from build123d import *

# Parameters (mm, degrees)
SKETCH_8_W               = 220
SKETCH_8_H               = 120
EXTRUDE_6_DEPTH          = 3
SKETCH_10_W              = 10
SKETCH_10_H              = 120
EXTRUDE_7_DEPTH          = 27
CUT_EXTRUDE_1_DEPTH      = 129.175660716
CUT_EXTRUDE_1_DEPTH_BACK = 129.175660716
SKETCH_9_R               = 2.05
SKETCH_11_R              = 3.6
CUT_EXTRUDE_2_DEPTH      = 25
CUT_EXTRUDE_4_DEPTH      = 129.175660716
CUT_EXTRUDE_4_DEPTH_BACK = 129.175660716
SKETCH_13_W              = 40
SKETCH_13_H              = 18.5
SKETCH_14_W              = 140
SKETCH_14_H              = 44
CUT_EXTRUDE_7_DEPTH      = 1
SKETCH_15_W              = 15
SKETCH_15_H              = 80
SKETCH_15_H_2            = 40
SKETCH_15_W_2            = 30
SKETCH_15_H_3            = 16
CUT_EXTRUDE_8_DEPTH      = 129.840987267
SKETCH_9_5_R             = 2
CUT_EXTRUDE_9_DEPTH      = 129.175660716
CUT_EXTRUDE_13_DEPTH     = 27
SKETCH_20_W              = 135
SKETCH_20_H              = 8
EXTRUDE_8_DEPTH          = 2
FILLET_1_R               = 3
FILLET_2_R               = 2


with BuildPart() as part:
    # Sketch 8 → Extrude 6 (new body)
    with BuildSketch(Plane(origin=(0, 0, 0), x_dir=(1, 0, 0), z_dir=(0, 1, 0))):
        Rectangle(SKETCH_8_W, SKETCH_8_H)
    extrude(amount=EXTRUDE_6_DEPTH)

    # Sketch 10 → Extrude 7 (add)
    with BuildSketch(Plane.XZ):
        with Locations((-105, 0)):
            Rectangle(SKETCH_10_W, SKETCH_10_H)
        with Locations((105, 0)):
            Rectangle(SKETCH_10_W, SKETCH_10_H)
    extrude(amount=EXTRUDE_7_DEPTH)

    # Sketch 9 → Cut-Extrude 1 (cut, two sides: drawn at the far end of the back side and taken through both)
    with BuildSketch(Plane(origin=(0, 0, 0), x_dir=(1, 0, 0), z_dir=(0, 1, 0)).offset(-CUT_EXTRUDE_1_DEPTH_BACK)):
        with Locations(Location((104.5, 54.5, 0), (0, 0, 270))):
            Circle(SKETCH_9_R)
        with Locations(Location((-104.5, 54.5, 0), (0, 0, 90))):
            Circle(SKETCH_9_R)
        with Locations(Location((-104.5, -54.5, 0), (0, 0, 270))):
            Circle(SKETCH_9_R)
        with Locations(Location((104.5, -54.5, 0), (0, 0, 90))):
            Circle(SKETCH_9_R)
    extrude(amount=CUT_EXTRUDE_1_DEPTH + CUT_EXTRUDE_1_DEPTH_BACK, mode=Mode.SUBTRACT)

    # Sketch 11 → Cut-Extrude 2 (cut)
    with BuildSketch(Plane(origin=(0, 3, 0), x_dir=(1, 0, 0), z_dir=(0, 1, 0))):
        with Locations(Location((-104.497380754, 54.5, 0), (0, 0, 270))):
            Circle(SKETCH_11_R)
        with Locations(Location((-104.497380754, -54.5, 0), (0, 0, 90))):
            Circle(SKETCH_11_R)
        with Locations(Location((104.5, -54.5, 0), (0, 0, 270))):
            Circle(SKETCH_11_R)
        with Locations(Location((104.5, 54.5, 0), (0, 0, 90))):
            Circle(SKETCH_11_R)
    extrude(amount=-CUT_EXTRUDE_2_DEPTH, mode=Mode.SUBTRACT)

    # Sketch 13 → Cut-Extrude 4 (cut, two sides: drawn at the far end of the back side and taken through both)
    with BuildSketch(Plane(origin=(0, 0, 0), x_dir=(0, 0, -1), z_dir=(1, 0, 0)).offset(-CUT_EXTRUDE_4_DEPTH_BACK)):
        with Locations((-25, -12.75)):
            Rectangle(SKETCH_13_W, SKETCH_13_H)
        with Locations((25, -12.75)):
            Rectangle(SKETCH_13_W, SKETCH_13_H)
    extrude(amount=CUT_EXTRUDE_4_DEPTH + CUT_EXTRUDE_4_DEPTH_BACK, mode=Mode.SUBTRACT)

    # Sketch 14 → Cut-Extrude 7 (cut)
    with BuildSketch(Plane(origin=(0, 3, 0), x_dir=(1, 0, 0), z_dir=(0, 1, 0))):
        Rectangle(SKETCH_14_W, SKETCH_14_H)
    extrude(amount=-CUT_EXTRUDE_7_DEPTH, mode=Mode.SUBTRACT)

    # Sketch 15 → Cut-Extrude 8 (cut, through all)
    with BuildSketch(Plane(origin=(0, 3, 0), x_dir=(1, 0, 0), z_dir=(0, 1, 0))):
        with Locations((-92.5, 0)):
            Rectangle(SKETCH_15_W, SKETCH_15_H)
        with Locations((92.5, 25)):
            Rectangle(SKETCH_15_W, SKETCH_15_H_2)
        Polygon((-44.702941459, -12), (44.702941459, -12), (0, -3.059411708), align=None)
        Polygon((-60, -8.940588292), (-60, 8.940588292), (-15.297058541, 0), align=None)
        Polygon((-44.702941459, 12), (44.702941459, 12), (0, 3.059411708), align=None)
        Polygon((60, -8.940588292), (60, 8.940588292), (15.297058541, 0), align=None)
        with Locations((0, -43)):
            Rectangle(SKETCH_15_W_2, SKETCH_15_H_3)
        with Locations((0, 43)):
            Rectangle(SKETCH_15_W_2, SKETCH_15_H_3)
        with Locations((92.5, -25)):
            Rectangle(SKETCH_15_W, SKETCH_15_H_2)
    extrude(amount=-CUT_EXTRUDE_8_DEPTH, mode=Mode.SUBTRACT)

    # Sketch 9_5 → Cut-Extrude 9 (cut, through all)
    with BuildSketch(Plane(origin=(0, 0, 0), x_dir=(1, 0, 0), z_dir=(0, 1, 0))):
        with Locations(Location((30, 28, 0), (0, 0, 270))):
            Circle(SKETCH_9_5_R)
        with Locations(Location((-30, 28, 0), (0, 0, 90))):
            Circle(SKETCH_9_5_R)
        with Locations(Location((30, -28, 0), (0, 0, 90))):
            Circle(SKETCH_9_5_R)
        with Locations(Location((-30, -28, 0), (0, 0, 270))):
            Circle(SKETCH_9_5_R)
    extrude(amount=CUT_EXTRUDE_9_DEPTH, mode=Mode.SUBTRACT)

    # Sketch 19 → Cut-Extrude 13 (cut)
    with BuildSketch(Plane.XZ.offset(27)):
        with BuildLine():
            Line((-100, 54.5), (-100, -54.5))
            ThreePointArc((-100, -54.5), (-101.318019485, -51.318019485), (-104.5, -50))
            Line((-104.5, -50), (-107, -50))
            Line((-107, -50), (-107, 50))
            Line((-107, 50), (-104.5, 50))
            ThreePointArc((-104.5, 50), (-101.318019485, 51.318019485), (-100, 54.5))
        make_face()
        with BuildLine():
            Line((100, 54.5), (100, -54.5))
            ThreePointArc((100, -54.5), (101.318019485, -51.318019485), (104.5, -50))
            Line((104.5, -50), (107, -50))
            Line((107, -50), (107, 50))
            Line((107, 50), (104.5, 50))
            ThreePointArc((104.5, 50), (101.318019485, 51.318019485), (100, 54.5))
        make_face()
    extrude(amount=-CUT_EXTRUDE_13_DEPTH, mode=Mode.SUBTRACT)

    # Sketch 20 → Extrude 8 (add)
    with BuildSketch(Plane.XZ):
        with Locations((0, 56)):
            Rectangle(SKETCH_20_W, SKETCH_20_H)
        with Locations((0, -56)):
            Rectangle(SKETCH_20_W, SKETCH_20_H)
        Polygon((-59, 32.5), (-39, 32.5), (-39, 29.5), (-54, 29.5), (-54, 25), (-59, 25), align=None)
        Polygon((54, 29.5), (39, 29.5), (39, 32.5), (59, 32.5), (59, 25), (54, 25), align=None)
        Polygon((59, -32.5), (39, -32.5), (39, -29.5), (54, -29.5), (54, -25), (59, -25), align=None)
        Polygon((-54, -29.5), (-39, -29.5), (-39, -32.5), (-59, -32.5), (-59, -25), (-54, -25), align=None)
    extrude(amount=EXTRUDE_8_DEPTH)

    # Fillet 1
    fillet_1_edges = [part.edges().sort_by_distance(p)[0] for p in [
        (-110, -12, -60),
        (110, -12, -60),
        (110, -12, 60),
        (-110, -12, 60),
    ]]
    fillet(fillet_1_edges, radius=FILLET_1_R)

    # Fillet 2
    fillet_2_edges = [part.edges().sort_by_distance(p)[0] for p in [
        (-108.5, -22, 45),
        (-108.5, -3.5, 45),
        (-108.5, -3.5, 5),
        (-108.5, -22, 5),
        (-108.5, -3.5, -5),
        (-108.5, -3.5, -45),
        (-108.5, -22, -45),
        (-108.5, -22, -5),
        (-85, 1.5, -40),
        (-100, 1.5, -40),
        (-85, 1.5, 40),
        (-100, 1.5, 40),
        (-15, 1.5, 51),
        (-15, 1.5, 35),
        (15, 1.5, 35),
        (15, 1.5, 51),
        (100, 1.5, 45),
        (85, 1.5, 5),
        (100, 1.5, 5),
        (15.297058541, 1, 0),
        (60, 1, -8.940588292),
        (60, 1, 8.940588292),
        (0, 1, -3.059411708),
        (-44.702941459, 1, -12),
        (44.702941459, 1, -12),
        (85, 1.5, -5),
        (100, 1.5, -5),
        (85, 1.5, -45),
        (100, 1.5, -45),
        (-15.297058541, 1, 0),
        (-60, 1, 8.940588292),
        (-60, 1, -8.940588292),
        (-15, 1.5, -35),
        (-15, 1.5, -51),
        (15, 1.5, -51),
        (15, 1.5, -35),
        (-44.702941459, 1, 12),
        (0, 1, 3.059411708),
        (44.702941459, 1, 12),
        (108.5, -3.5, 45),
        (108.5, -22, 45),
        (108.5, -3.5, 5),
        (108.5, -22, 5),
        (108.5, -3.5, -45),
        (108.5, -3.5, -5),
        (108.5, -22, -45),
        (108.5, -22, -5),
        (-107, 0, 0),
        (107, 0, 0),
    ]]
    fillet(fillet_2_edges, radius=FILLET_2_R)


solid = part.part
Can you work these out from the model? Positions are in its coordinate system, mm. A direction names the side the tool comes from. Round coordinates to 2 decimals unless told otherwise and drop trailing zeros. Loops run counter-clockwise (first coordinate to the right, second up) from the corner with the lowest first, then second, coordinate; pieces in that order, holes last. Notation, with made-up numbers: (-14.75, -9.75) - (16.25, -9.75) arc R24 ccw to (16.25, 19.25) - close; hole circle Ø5 at (66.5, 17.5). An arc over 180 degrees is marked (long way). Use CSV: the item, a comma, the result in double quotes. Start each with the question number.
1) We'd pull the mould along X, two halves only. Please class faces 1 (the flat face through (-110, -12, -1)), 2 (the flat face through (-2, 3, -28)), 3 (the flat face through (-51, -2, 30)): released by +X, released by -X, zero draft, split by the parting line, or undercut.
2) If we section it at B-B on z = 16.5: Count the separate pieces of the cut face and the enclosed holes in it, plus the area to 3 significant figures.
3) For pin 1 Ø6.5 at (x, z) = (-104.5, 54.5) entering from +Y; pin 2 Ø1.5 at (y, z) = (-21, 31) entering from -X; pin 3 Ø6 at (x, z) = (-19, -28.5) entering from -Y, each with a flat end and sliding along its axis, tell me the tip position at first contact or that it passes through.
4) Please list where these lines run through material, in increasing order: probe 1 along X at (y, z) = (1.25, -15); probe 2 along X at (y, z) = (-25.55, 54.5); probe 3 along Z at (x, y) = (-104.5, -23.85). Write a range as [from, to].
5) If we section it at C-C on x = -95: Write out the boundary of the cut face in (y, z).
6) If we section it at A-A on y = -24.75: Write out the boundary of the cut face in (x, z), plus the area to 3 significant figures.
7) For faces 4 (the flat face through (107.2, -27, 0.8)), 5 (the flat face through (-100, -13, -57)), 6 (the flat face through (12.816, 1.014, -5.623)), 7 (the cylindrical face through (-107.53, -9.32, 52.56)), 8 (the cylindrical face through (-101.283, -13.689, -51.353)), which set-ups out of +Z, -Z, +X, -X, +Y, -Y let a thin tool reach every point of the face, with its end or its side?
Geometry results:
1,face 1,"released by -X"
1,face 2,"zero draft"
1,face 3,"undercut"
2,separate pieces,"5"
2,enclosed holes,"0"
2,area,"483 mm2"
3,pin 1,"stops at y = -22"
3,pin 2,"passes through"
3,pin 3,"stops at y = 0"
4,probe 1,"x = [-110, -100], [-85, 85], [100, 110]"
4,probe 2,"x = [-110, -106.55], [-102.45, -100], [100, 102.45], [106.55, 110]"
4,probe 3,"z = [-60, -56.55], [-52.45, -50], [50, 52.45], [56.55, 60]"
5,outline,"(0, -60) - (3, -60) - (3, -40) - (0, -40) - close; (0, 40) - (3, 40) - (3, 60) - (0, 60) - close"
6,outline,"(-110, -57) arc R3 ccw to (-107, -60) - (-100, -60) - (-100, -54.5) arc R4.5 ccw to (-104.5, -50) - (-107, -50) - (-107, 50) - (-104.5, 50) arc R4.5 ccw to (-100, 54.5) - (-100, 60) - (-107, 60) arc R3 ccw to (-110, 57) - close; (100, -60) - (107, -60) arc R3 ccw to (110, -57) - (110, 57) arc R3 ccw to (107, 60) - (100, 60) - (100, 54.5) arc R4.5 ccw to (104.5, 50) - (107, 50) - (107, -50) - (104.5, -50) arc R4.5 ccw to (100, -54.5) - close; hole circle Ø4.1 at (-104.5, -54.5); hole circle Ø4.1 at (-104.5, 54.5); hole circle Ø4.1 at (104.5, -54.5); hole circle Ø4.1 at (104.5, 54.5)"
6,area,"922 mm2"
7,face 4,"+Z, -Z, +X, -X, -Y"
7,face 5,"+Z, -Z, -Y"
7,face 6,"+Y, -Y"
7,face 7,"+Y"
7,face 8,"-Y"
